Input: part model. Units: mm. Frame: model coordinates. Give positions to 0.01 mm unless a question says otherwise; leave off trailing zeros. Loops run counter-clockwise (first coordinate to the right, second up) from the corner with the lowest first, then second, coordinate; pieces in that order, holes last. Notation, with made-up numbers: (88, -18) -> (137, -18) arc R30 ccw to (137, 9) -> close; hole circle Ø9 at (75.5, -38). An arc over 180 degrees is marked (long way). Use CSV: the item, a comma, the result in double quotes.
```python
from build123d import *

# Parameters (mm, degrees)
SKETCH2_R          = 2.625
SKETCH2_R_2        = 3.125
MAINPLATE_DEPTH    = 6.5
PRESSFITNUTS_DEPTH = 5
CUT_EXTRUDE2_DEPTH = 6.5
FILLET2_R          = 10


with BuildPart() as part:
    # Sketch2 → MainPlate (new body)
    with BuildSketch(Plane(origin=(0, 0, 0), x_dir=(1, 0, 0), z_dir=(0, 1, 0))):
        with BuildLine():
            Line((24.899900609, -92.429929219), (0.2, -92.5))
            Line((0.2, -92.5), (-24.5, -92.5))
            ThreePointArc((-24.5, -92.5), (-27.871368271, -92.016678166), (-30.971160559, -90.605645997))
            Line((-30.971160559, -90.605645997), (-99.683475736, -46.605645997))
            ThreePointArc((-99.683475736, -46.605645997), (-104.578950448, -40.347025165), (-104.490786491, -32.401697323))
            Line((-104.490786491, -32.401697323), (-83.778471314, 24.598302677))
            ThreePointArc((-83.778471314, 24.598302677), (-80.773721892, 29.191692934), (-76.037940173, 31.966602781))
            Line((-76.037940173, 31.966602781), (-24.911380811, 47.741345462))
            ThreePointArc((-24.911380811, 47.741345462), (-22.845839779, 48.308813352), (-20.712315177, 48.5))
            Line((-20.712315177, 48.5), (0, 48.5))
            Line((0, 48.5), (20.712231832, 48.558758223))
            ThreePointArc((20.712231832, 48.558758223), (22.846290221, 48.373624884), (24.913432777, 47.812018957))
            Line((24.913432777, 47.812018957), (76.084537362, 32.182379345))
            ThreePointArc((76.084537362, 32.182379345), (80.828172093, 29.420915478), (83.845940292, 24.836067799))
            Line((83.845940292, 24.836067799), (104.719873926, -32.104944614))
            ThreePointArc((104.719873926, -32.104944614), (104.830577421, -40.049990373), (99.952877324, -46.322473865))
            Line((99.952877324, -46.322473865), (31.365661085, -90.517224974))
            ThreePointArc((31.365661085, -90.517224974), (28.26988419, -91.937045184), (24.899900609, -92.429929219))
        make_face()
        with Locations(Location((-72.5, 20.5, 0), (0, 0, 90))):
            Circle(SKETCH2_R, mode=Mode.SUBTRACT)
        with Locations(Location((-20.712315177, 36.5, 0), (0, 0, 90))):
            Circle(SKETCH2_R, mode=Mode.SUBTRACT)
        with Locations(Location((-93.212315177, -36.5, 0), (0, 0, 90))):
            Circle(SKETCH2_R, mode=Mode.SUBTRACT)
        with Locations(Location((-58.856157589, -58.5, 0), (0, 0, 90))):
            Circle(SKETCH2_R, mode=Mode.SUBTRACT)
        with Locations(Location((-24.5, -80.5, 0), (0, 0, 90))):
            Circle(SKETCH2_R, mode=Mode.SUBTRACT)
        with Locations(Location((-24.5, -36.5, 0), (0, 0, 90))):
            Circle(SKETCH2_R, mode=Mode.SUBTRACT)
        with Locations(Location((-72.5, -22.5, 0), (0, 0, 90))):
            Circle(SKETCH2_R, mode=Mode.SUBTRACT)
        with Locations(Location((24.74103568, -36.430154559, 0), (0, 0, 90))):
            Circle(SKETCH2_R, mode=Mode.SUBTRACT)
        with Locations(Location((24.865858124, -80.429977506, 0), (0, 0, 90))):
            Circle(SKETCH2_R, mode=Mode.SUBTRACT)
        with Locations(Location((59.159466244, -58.332601952, 0), (0, 0, 90))):
            Circle(SKETCH2_R, mode=Mode.SUBTRACT)
        with Locations(Location((93.453074364, -36.235226398, 0), (0, 0, 90))):
            Circle(SKETCH2_R, mode=Mode.SUBTRACT)
        with Locations(Location((72.701126299, -22.294040956, 0), (0, 0, 90))):
            Circle(SKETCH2_R, mode=Mode.SUBTRACT)
        with Locations(Location((72.579140729, 20.705786015, 0), (0, 0, 90))):
            Circle(SKETCH2_R, mode=Mode.SUBTRACT)
        with Locations(Location((20.746274317, 36.55880651, 0), (0, 0, 90))):
            Circle(SKETCH2_R, mode=Mode.SUBTRACT)
        with Locations(Location((0, -36.5, 0), (0, 0, 90))):
            Circle(SKETCH2_R_2, mode=Mode.SUBTRACT)
        with Locations(Location((0.182929062, -80.464988753, 0), (0, 0, 90))):
            Circle(SKETCH2_R_2, mode=Mode.SUBTRACT)
        with Locations(Location((0.103546099, -24.5, 0), (0, 0, 90))):
            Circle(SKETCH2_R, mode=Mode.SUBTRACT)
        with BuildLine():
            Line((2.580926866, 27.523084214), (2.668870128, 17.523084214))
            ThreePointArc((2.668870128, 17.523084214), (0.067055845, 14.875101503), (-2.580926866, 17.476915786))
            Line((-2.580926866, 17.476915786), (-2.668870128, 27.476915786))
            ThreePointArc((-2.668870128, 27.476915786), (-0.067055845, 30.124898497), (2.580926866, 27.523084214))
        make_face(mode=Mode.SUBTRACT)
    extrude(amount=MAINPLATE_DEPTH)

    # Sketch8 → PressFitNuts (cut)
    with BuildSketch(Plane(origin=(0, 6.5, 0), x_dir=(1, 0, 0), z_dir=(0, 1, 0))):
        Polygon((-3.847658971, -26.891926384), (0.199412577, -29.117807158), (4.150617647, -26.725880774), (4.054751169, -22.108073616), (0.007679621, -19.882192842), (-3.943525449, -22.274119226), align=None)
        Polygon((-19.881197846, -36.5), (-22.190598923, -32.5), (-26.809401077, -32.5), (-29.118802154, -36.5), (-26.809401077, -40.5), (-22.190598923, -40.5), align=None)
        Polygon((-67.881197846, -22.5), (-70.190598923, -18.5), (-74.809401077, -18.5), (-77.118802154, -22.5), (-74.809401077, -26.5), (-70.190598923, -26.5), align=None)
        Polygon((-67.881197846, 20.5), (-70.190598923, 24.5), (-74.809401077, 24.5), (-77.118802154, 20.5), (-74.809401077, 16.5), (-70.190598923, 16.5), align=None)
        Polygon((-88.593513024, -36.5), (-90.9029141, -32.5), (-95.521716254, -32.5), (-97.831117331, -36.5), (-95.521716254, -40.5), (-90.9029141, -40.5), align=None)
        Polygon((-54.237355435, -58.5), (-56.546756512, -54.5), (-61.165558665, -54.5), (-63.474959742, -58.5), (-61.165558665, -62.5), (-56.546756512, -62.5), align=None)
        Polygon((-24.5, -75.881197846), (-28.5, -78.190598923), (-28.5, -82.809401077), (-24.5, -85.118802154), (-20.5, -82.809401077), (-20.5, -78.190598923), align=None)
        Polygon((-16.093513024, 36.5), (-18.4029141, 40.5), (-23.021716254, 40.5), (-25.331117331, 36.5), (-23.021716254, 32.5), (-18.4029141, 32.5), align=None)
        Polygon((18.448230028, 32.552271126), (16.127490749, 36.545703551), (18.425535038, 40.552238935), (23.044318606, 40.565341893), (25.365057885, 36.571909468), (23.067013596, 32.565374085), align=None)
        Polygon((20.859322741, -78.131933217), (24.852755166, -75.811193938), (28.859290549, -78.109238227), (28.872393508, -82.728021795), (24.878961083, -85.048761074), (20.872425699, -82.750716785), align=None)
        Polygon((56.861421955, -62.339137336), (54.540682676, -58.34570491), (56.838726965, -54.339169527), (61.457510533, -54.326066569), (63.778249812, -58.319498994), (61.480205523, -62.326034377), align=None)
        Polygon((91.155030075, -40.241761781), (88.834290796, -36.248329356), (91.132335085, -32.241793973), (95.751118653, -32.228691014), (98.071857931, -36.222123439), (95.773813642, -40.228658823), align=None)
        Polygon((70.28109644, 16.699250632), (67.960357161, 20.692683057), (70.25840145, 24.69921844), (74.877185018, 24.712321399), (77.197924297, 20.718888974), (74.899880008, 16.71235359), align=None)
        Polygon((70.40308201, -26.300576339), (68.082342731, -22.307143914), (70.38038702, -18.300608531), (74.999170588, -18.287505572), (77.319909867, -22.280937997), (75.021865578, -26.287473381), align=None)
        Polygon((22.442991391, -40.436689943), (20.122252112, -36.443257518), (22.420296401, -32.436722134), (27.039079969, -32.423619176), (29.359819248, -36.417051601), (27.061774959, -40.423586984), align=None)
    extrude(amount=-PRESSFITNUTS_DEPTH, mode=Mode.SUBTRACT)

    # Sketch11 → Cut-Extrude2 (cut)
    with BuildSketch(Plane(origin=(0, 0, 0), x_dir=(1, 0, 0), z_dir=(0, 1, 0))):
        with BuildLine():
            Line((-111.9, 4.5), (-111.9, -116.15))
            Line((-111.9, -116.15), (-86.5, -116.15))
            Line((-86.5, -116.15), (-36.5, -116.15))
            Line((-36.5, -116.15), (-36.5, -59))
            ThreePointArc((-36.5, -59), (-42.357864376, -44.857864376), (-56.5, -39))
            Line((-56.5, -39), (-66.5, -39))
            ThreePointArc((-66.5, -39), (-80.642135624, -33.142135624), (-86.5, -19))
            Line((-86.5, -19), (-86.5, 4.5))
            Line((-86.5, 4.5), (-86.5, 44.576396133))
            Line((-86.5, 44.576396133), (-111.9, 44.576396133))
            Line((-111.9, 44.576396133), (-111.9, 4.5))
        make_face()
        with BuildLine():
            Line((86.5, 4.5), (86.5, 44.576396133))
            Line((86.5, 44.576396133), (111.9, 44.576396133))
            Line((111.9, 44.576396133), (111.9, 4.5))
            Line((111.9, 4.5), (111.9, -116.15))
            Line((111.9, -116.15), (86.5, -116.15))
            Line((86.5, -116.15), (36.5, -116.15))
            Line((36.5, -116.15), (36.5, -59))
            ThreePointArc((36.5, -59), (42.357864376, -44.857864376), (56.5, -39))
            Line((56.5, -39), (66.5, -39))
            ThreePointArc((66.5, -39), (80.642135624, -33.142135624), (86.5, -19))
            Line((86.5, -19), (86.5, 4.5))
        make_face()
    extrude(amount=CUT_EXTRUDE2_DEPTH, mode=Mode.SUBTRACT)

    # Fillet2
    fillet2_edges = [part.edges().sort_by_distance(p)[0] for p in [
        (36.5, 3.25, 87.208870401),
        (-36.5, 3.25, 87.065248111),
    ]]
    fillet(fillet2_edges, radius=FILLET2_R)


solid = part.part
```
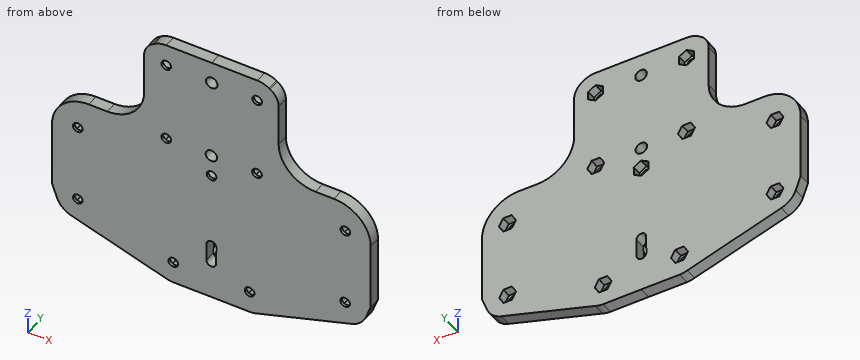
1) Ray query, line 1 (X direction, y = 0.95, z = 80.5) (3 decimals); line 2 (X direction, y = 2.5, z = 25); line 3 (Z direction, x = -74, y = 0.75). Return the intervals inside material, ascending.
From the geometry:
line 1,"x = -36.5 to -27.125, -21.875 to -2.942, 3.308 to 22.242, 27.49 to 36.5"
line 2,"x = -85.58 to -75.68, -69.32 to -3.89, 4.11 to 69.65, 75.76 to 85.58"
line 3,"z = -32.6 to -22.65, -18.35 to 20.35, 24.65 to 37.54"
2) Section query D-D (x = -43). Return loops of the section in (y, z).
From the geometry:
outline,"(0, -42.16) -> (6.5, -42.16) -> (6.5, 44.24) -> (0, 44.24) -> close"
3) Contact query for flat-ended pins moving along their axis: pin 1 (4 mm diameter, centred on x = -72, z = -20, fed in from +Y); pin 2 (2 mm diameter, centred on x = 63.5, y = 2.5, fed in from +Z); pin 3 (3.5 mm diameter, centred on y = 4, z = 80, fed in from +X). Output: stop coordinate, or through.
From the geometry:
pin 1,"stops at y = 1.5"
pin 2,"stops at z = 39"
pin 3,"stops at x = 36.5"
4) Section query A-A (x = -72.5). Return loops of the section in (y, z) (3 decimals), then the cut area to 3 significant figures.
From the geometry:
outline,"(0, -33.058) -> (6.5, -33.058) -> (6.5, -24.5) -> (1.5, -24.5) -> (1.5, -23.125) -> (0, -23.125) -> close; (0, -17.875) -> (1.5, -17.875) -> (1.5, -16.5) -> (6.5, -16.5) -> (6.5, 18.5) -> (1.5, 18.5) -> (1.5, 19.875) -> (0, 19.875) -> close; (0, 25.125) -> (1.5, 25.125) -> (1.5, 26.5) -> (6.5, 26.5) -> (6.5, 38.079) -> (0, 38.079) -> close"
area,"367 mm^2"
5) Section query C-C (z = 48.5). Return loops of the section in (x, y), then the cut area to 3 significant figures.
From the geometry:
outline,"(-39.48, 0) -> (39.48, 0) -> (39.48, 6.5) -> (-39.48, 6.5) -> close"
area,"513 mm^2"
6) Section query B-B (y = 5.5). Give the number of separate pieces and of enclosed holes in the cut face, then the cut area to 3 significant figures.
From the geometry:
separate pieces,"1"
enclosed holes,"14"
area,"16,900 mm^2"
